Autodesk Inventor part; units mm, degrees
ref_plane "YZ Plane" through (0, 0, 0) normal (1, 0, 0) x (0, 1, 0)
ref_plane "XZ Plane" through (0, 0, 0) normal (0, 1, 0) x (-1, 0, 0)
ref_plane "XY Plane" through (0, 0, 0) normal (0, 0, 1) x (1, 0, 0)
sketch "Sketch2" plane through (0, 0, 0) normal (0, 0, 1) x (1, 0, 0)
  line L0 (-50, -100) -> (50, -100)
  line L1 (50, -100) -> (50, 100)
  line L2 (50, 100) -> (-50, 100)
  line L3 (-50, 100) -> (-50, -100)
  line L4 (-50, -100) -> (50, 100) construction
  line L5 (50, -100) -> (-50, 100) construction
  line L6 (-100, -150) -> (100, -150)
  line L7 (100, -150) -> (100, 150)
  line L8 (100, 150) -> (-100, 150)
  line L9 (-100, 150) -> (-100, -150)
  point P0 (0, 0)
  dimension "d29" = 100
  dimension "d30" = 200
  dimension "d31" = 50
extrude "Plate2" add sketch "Sketch2" along normal blind 10
sketch "Sketch5" plane through (0, 0, 10) normal (0, 0, 1) x (1, 0, 0)
  line L0 (50, 100) -> (50, -100) construction
  line L1 (50, -100) -> (-50, -100) construction
  line L2 (-50, -100) -> (-50, 100) construction
  line L3 (-50, 100) -> (50, 100) construction
  line L4 (100, -150) -> (-100, -150) construction
  line L5 (100, 150) -> (100, -150) construction
  line L6 (-100, 150) -> (100, 150) construction
  line L7 (-100, -150) -> (-100, 150) construction
  line L8 (-81, 131) -> (81, 131) construction
  line L9 (81, 131) -> (81, -131) construction
  line L10 (81, -131) -> (-81, -131) construction
  line L11 (-81, -131) -> (-81, 131) construction
  circle A0 centre (-81, -131) radius 8.5
  circle A1 centre (-81, 131) radius 8.5
  circle A2 centre (-81, 0) radius 8.5
  circle A3 centre (-81, -65.5) radius 8.5
  circle A4 centre (-81, 65.5) radius 8.5
  line L12 (-50, 0) -> (50, 0) construction
  circle A5 centre (-27, -131) radius 8.5
  circle A6 centre (-27, -65.5) radius 8.5
  circle A7 centre (-27, 0) radius 8.5
  circle A8 centre (-27, 65.5) radius 8.5
  circle A9 centre (-27, 131) radius 8.5
  circle A10 centre (27, -131) radius 8.5
  circle A11 centre (27, -65.5) radius 8.5
  circle A12 centre (27, 0) radius 8.5
  circle A13 centre (27, 65.5) radius 8.5
  circle A14 centre (27, 131) radius 8.5
  circle A15 centre (81, -131) radius 8.5
  circle A16 centre (81, -65.5) radius 8.5
  circle A17 centre (81, 0) radius 8.5
  circle A18 centre (81, 65.5) radius 8.5
  circle A19 centre (81, 131) radius 8.5
  point P0 (0, 0)
  point P1 (0, -131)
  dimension "d33" = 17
  dimension "d34" = 19
  dimension "d35" = 65.5
  dimension "d36" = 65.5
  dimension "d39" = 54
extrude "Cut3" cut sketch "Sketch5" against normal blind 10
fillet "Corner Round1" radius 6 8 edges at (-100, -150, 5) (-100, 150, 5) (100, 150, 5) (100, -150, 5) (50, -100, 5) (-50, -100, 5) (-50, 100, 5) (50, 100, 5)
equation "\"d35\" = d36"
equation "\"d44\" = Thickness"
equation "\"d14\" = Thickness"
equation "\"BendReliefDepth\" = 0.5 * Thickness"
equation "\"TransitionRadius\" = BendRadius"
equation "\"JacobiRadiusSize\" = BendRadius"
properties part number "PRS 9606 charging flange round_1200" material "Steel"
Model file for the job. Use its own axes, mm. A direction names the side the tool comes from. Round coordinates to 2 decimals unless told otherwise and drop trailing zeros. Order: outer loops, then holes, each group sorted by start corner. A loop starts at its lowest first (then second) coordinate and runs counter-clockwise, first axis right, second up.
(1) Band-saw the part on D-D (z = 6). Give the number of separate pieces and of enclosed holes in the cut face, then the cut area to 3 significant figures.
(2) Band-saw the part on A-A (x = -27). List the corners of the cut face in (y, z).
(3) Drill centre lines: line 1 (Y direction, x = -81, z = 4); line 2 (Y direction, x = -27, z = 2); line 3 (X direction, y = -49, z = 5). Where is each one in solid material? Low to high.
(4) Pull direction Y, two halves, no side cores. Call faces 3 (the face through (-23.08, -138.54, 5.07)), 4 (the face through (98.196, -148.289, 5.07)), 5 (the face through (-89.49, -65.13, 5.07)), 6 (the face through (-100, 2, 5)): released by +Y, released by -Y, zero draft, split by the parting line, or undercut.
(5) Band-saw the part on C-C (y = 0). List the corners of the cut face in (x, z), then the cut area to 3 significant figures.
(6) 3-axis set-ups, long thin cutter, end or side, ignore diameter. For faces 1 (the face through (-1, -150, 5)), 2 (the face through (-50, 1, 5)): which of +Z, -Z, +X, -X, +Y, -Y reach the whole face in a straight line?
(7) Band-saw the part on B-B (x = 81). List the corners of the cut face in (y, z).
(8) Pin check, flat tip, straight feed: pin 1 (15.5 mm diameter, centred on x = 81, y = 0, fed in from -Z). Stop position of the tip, or through.
Verdict:
1. separate pieces: 1
1. enclosed holes: 15
1. area: 36,800 mm2
2. outline: (-150, 0) - (-139.5, 0) - (-139.5, 10) - (-150, 10) - close; (-122.5, 0) - (-100, 0) - (-100, 10) - (-122.5, 10) - close; (100, 0) - (122.5, 0) - (122.5, 10) - (100, 10) - close; (139.5, 0) - (150, 0) - (150, 10) - (139.5, 10) - close
3. line 1: y = -150 to -139.5, -122.5 to -74, -57 to -8.5, 8.5 to 57, 74 to 122.5, 139.5 to 150
3. line 2: y = -150 to -139.5, -122.5 to -100, 100 to 122.5, 139.5 to 150
3. line 3: x = -100 to -50, 50 to 100
4. face 3: undercut
4. face 4: released by -Y
4. face 5: undercut
4. face 6: zero draft
5. outline: (-100, 0) - (-89.5, 0) - (-89.5, 10) - (-100, 10) - close; (-72.5, 0) - (-50, 0) - (-50, 10) - (-72.5, 10) - close; (50, 0) - (72.5, 0) - (72.5, 10) - (50, 10) - close; (89.5, 0) - (100, 0) - (100, 10) - (89.5, 10) - close
5. area: 660 mm2
6. face 1: +Z, -Z, +X, -X, -Y
6. face 2: +Z, -Z
7. outline: (-150, 0) - (-139.5, 0) - (-139.5, 10) - (-150, 10) - close; (-122.5, 0) - (-74, 0) - (-74, 10) - (-122.5, 10) - close; (-57, 0) - (-8.5, 0) - (-8.5, 10) - (-57, 10) - close; (8.5, 0) - (57, 0) - (57, 10) - (8.5, 10) - close; (74, 0) - (122.5, 0) - (122.5, 10) - (74, 10) - close; (139.5, 0) - (150, 0) - (150, 10) - (139.5, 10) - close
8. pin 1: passes through
